Here's how the part is built. I have some questions about the finished solid (model axes, mm). Give positions to 0.01 mm unless a question says otherwise; leave off trailing zeros. Write each loop counter-clockwise with the first axis right and the second up, starting at its lowest first coordinate (ties: lowest second). Pieces come first, ordered by that corner, then holes. Notation, with made-up numbers: (67, -14.75) -> (93, -14.75) arc R25 ccw to (93, 9.25) -> close; hole circle Ø9 at (40.25, 34.25). An arc over 180 degrees is marked (long way). Answer as CSV lines item,"result". Start each with the question number.
from build123d import *

# Parameters (mm, degrees)
BOSS_EXTRUDE3_DEPTH     = 7.5
CUT_EXTRUDE4_DEPTH      = 1.5
BOSS_EXTRUDE5_DEPTH     = 1.5
SKETCH4_R               = 3
BEARING_HOLE_DEPTH      = 1.25
SHAFT_HOLE_DEPTH        = 33.837885572
SHAFT_HOLE_DEPTH_BACK   = 2.5
SKETCH7_R               = 1.5
CUT_EXTRUDE6_DEPTH      = 178.77712661
CUT_EXTRUDE6_DEPTH_BACK = 178.77712661
SKETCH8_R               = 1.5


with BuildPart() as part:
    # Sketch1 → Boss-Extrude3 (new, symmetric)
    with BuildSketch(Plane.XY):
        with BuildLine():
            Line((-157.569240482, 27.783708427), (-172.341356777, 30.388431092))
            ThreePointArc((-172.341356777, 30.388431092), (-175, 0), (-172.341356777, -30.388431092))
            Line((-172.341356777, -30.388431092), (-157.569240482, -27.783708427))
            ThreePointArc((-157.569240482, -27.783708427), (-160, 0), (-157.569240482, 27.783708427))
        make_face()
    extrude(amount=BOSS_EXTRUDE3_DEPTH, both=True)

    # Sketch1_6 → Cut-Extrude4 (cut, symmetric)
    with BuildSketch(Plane.XY):
        with BuildLine():
            Line((-157.569240482, 27.783708427), (-172.341356777, 30.388431092))
            ThreePointArc((-172.341356777, 30.388431092), (-175, 0), (-172.341356777, -30.388431092))
            Line((-172.341356777, -30.388431092), (-157.569240482, -27.783708427))
            ThreePointArc((-157.569240482, -27.783708427), (-160, 0), (-157.569240482, 27.783708427))
        make_face()
    extrude(amount=CUT_EXTRUDE4_DEPTH, both=True, mode=Mode.SUBTRACT)


with BuildPart() as cut_extrude4_piece_1:
    # of the separate pieces the step leaves, piece 1, a body of its own (cut_extrude4_pieces)
    add(part.part.solids().sort_by_distance((-172.341356777, 30.388431092, -1.5))[0])



with BuildPart() as cut_extrude4_piece_2:
    # of the separate pieces the step leaves, piece 2, a body of its own (cut_extrude4_pieces)
    add(part.part.solids().sort_by_distance((-172.341356777, 30.388431092, 7.5))[0])


with BuildPart() as cut_extrude4_piece_1_1:
    add(cut_extrude4_piece_1.part)

    add(cut_extrude4_piece_2.part)  # Boss-Extrude5 merges Cut-Extrude4 piece 2
    # Sketch6 → Boss-Extrude5 (add, symmetric)
    with BuildSketch(Plane.XY):
        with BuildLine():
            Line((-159.824122084, 7.5), (-174.839211849, 7.5))
            ThreePointArc((-174.839211849, 7.5), (-175, 0), (-174.839211849, -7.5))
            Line((-174.839211849, -7.5), (-159.824122084, -7.5))
            ThreePointArc((-159.824122084, -7.5), (-160, 0), (-159.824122084, 7.5))
        make_face()
    extrude(amount=BOSS_EXTRUDE5_DEPTH, both=True)

    # Sketch4 → bearing hole (cut, symmetric)
    with BuildSketch(Plane(origin=(-167.5, 0, 0), x_dir=(0, 0, -1), z_dir=(1, 0, 0))):
        Circle(SKETCH4_R)
    extrude(amount=BEARING_HOLE_DEPTH, both=True, mode=Mode.SUBTRACT)

    # Sketch7 → shaft hole (cut, two sides: drawn at the far end of the back side and taken through both)
    with BuildSketch(Plane(origin=(-167.5, 0, 0), x_dir=(0, 0, -1), z_dir=(1, 0, 0)).offset(-SHAFT_HOLE_DEPTH_BACK)):
        with Locations(Location((0, 0, 0), (0, 0, 180))):
            Circle(SKETCH7_R)
    extrude(amount=SHAFT_HOLE_DEPTH + SHAFT_HOLE_DEPTH_BACK, mode=Mode.SUBTRACT)

    # Sketch8 → Cut-Extrude6 (cut, two sides: drawn at the far end of the back side and taken through both)
    with BuildSketch(Plane.XY.offset(-CUT_EXTRUDE6_DEPTH_BACK)):
        with Locations((-166.306502189, 19.95989303)):
            Circle(SKETCH8_R)
        with Locations((-167.201226072, 10)):
            Circle(SKETCH8_R)
        with Locations((-167.201226072, -10)):
            Circle(SKETCH8_R)
        with Locations((-166.306502189, -19.95989303)):
            Circle(SKETCH8_R)
    extrude(amount=CUT_EXTRUDE6_DEPTH + CUT_EXTRUDE6_DEPTH_BACK, mode=Mode.SUBTRACT)


solid = cut_extrude4_piece_1_1.part
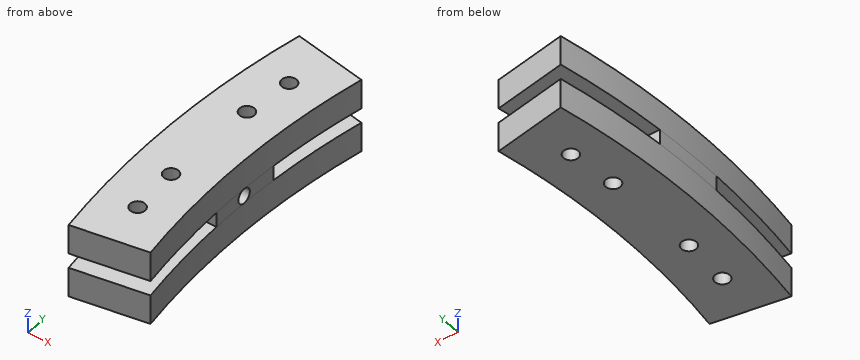
Item 1: If we section it at B-B (z = 0): Please give me the cut outline in (x, y).
Item 2: If we section it at A-A (y = -10): Please give me the cut outline in (x, z).
Item 3: I'm going to push flat-ended pins straight in: pin 1 (2.5 mm diameter, centred on x = -166.31, y = -19.96, fed in from -Z); pin 2 (8 mm diameter, centred on y = -9, z = 3.5, fed in from +X); pin 3 (5 mm diameter, centred on y = -11, z = -3, fed in from -X); pin 4 (4 mm diameter, centred on y = 0, z = 0, fed in from +X). Where does each tip first touch, or does it pass through?
Item 4: If we section it at C-C (x = -163.75): Please give me the cut outline in (y, z).
Item 5: If I drill on line 1 (Z direction, x = -170.75, y = -15.5); line 2 (Y direction, x = -165.5, z = -5), over which ranges is the centre line in solid material (lowest first)? Write a range as [from, to].
Item 6: If we section it at D-D (z = 6.75): Please give me the cut outline in (x, y), and give its area (3 significant figures).
Final values:
1,outline,"(-174.84, -7.5) -> (-159.82, -7.5) arc R160 cw to (-159.99, -1.5) -> (-166.25, -1.5) -> (-166.25, -3) -> (-168.75, -3) -> (-168.75, -1.5) -> (-170, -1.5) -> (-170, 1.5) -> (-168.75, 1.5) -> (-168.75, 3) -> (-166.25, 3) -> (-166.25, 1.5) -> (-159.99, 1.5) arc R160 cw to (-159.82, 7.5) -> (-174.84, 7.5) arc R175 ccw to start"
2,outline,"(-174.71, -7.5) -> (-168.7, -7.5) -> (-168.7, -1.5) -> (-174.71, -1.5) -> close; (-174.71, 1.5) -> (-168.7, 1.5) -> (-168.7, 7.5) -> (-174.71, 7.5) -> close; (-165.7, -7.5) -> (-159.69, -7.5) -> (-159.69, -1.5) -> (-165.7, -1.5) -> close; (-165.7, 1.5) -> (-159.69, 1.5) -> (-159.69, 7.5) -> (-165.7, 7.5) -> close"
3,pin 1,"through"
3,pin 2,"x = -159.47"
3,pin 3,"x = -174.79"
3,pin 4,"x = -159.99"
4,outline,"(-28.87, -7.5) -> (28.87, -7.5) -> (28.87, -1.5) -> (7.5, -1.5) -> (7.5, 1.5) -> (28.87, 1.5) -> (28.87, 7.5) -> (-28.87, 7.5) -> (-28.87, 1.5) -> (-7.5, 1.5) -> (-7.5, -1.5) -> (-28.87, -1.5) -> close; hole circle Ø3 at (0, 0)"
5,line 1,"[-7.5, -1.5], [1.5, 7.5]"
5,line 2,"[-29.18, -21.22], [-18.7, 18.7], [21.22, 29.18]"
6,outline,"(-172.34, -30.39) -> (-157.57, -27.78) arc R160 cw to (-157.57, 27.78) -> (-172.34, 30.39) arc R175 ccw to start; hole circle Ø3 at (-167.2, -10); hole circle Ø3 at (-167.2, 10); hole circle Ø3 at (-166.31, -19.96); hole circle Ø3 at (-166.31, 19.96)"
6,area,"849 mm2"
